Check sheet for the modelled part. Datum: model origin and axes. Units: mm. Face numbers are marked on the shaded views. Round coordinates to 2 decimals unless told otherwise and drop trailing zeros. Order: outer loops, then holes, each group sorted by start corner. A loop starts at its lowest first (then second) coordinate and runs counter-clockwise, first axis right, second up. Notation, with made-up numbers: M 53.25,-17.5 L 83.25,-17.5 A7 ccw 83.25,-8.5 Z; hole C -30,66.5 d3. An arc over 180 degrees is marked long. One line per item, written item: value. Start each with the question number.
(1) Release check for a two-part mould opening along Y. For the marked faces 1, 2 and 3 record: released by +Y, released by -Y, zero draft, split by the parting line, or undercut.
(2) Cross-section at B-B, the plane y = 31. Enter the section's corners in (x, z), and give its area (3 significant figures).
(3) Thickness scan on L1, parallel to Z at x = 0.05, y = 2; L2, parallel to Z at x = 0.4, y = 19.5; L3, parallel to X at y = 31.5, z = -0.35. Record the ranges inside material, lowest first.
(4) Cross-section at A-A, the plane y = 25. Enter the section's corners in (x, z).
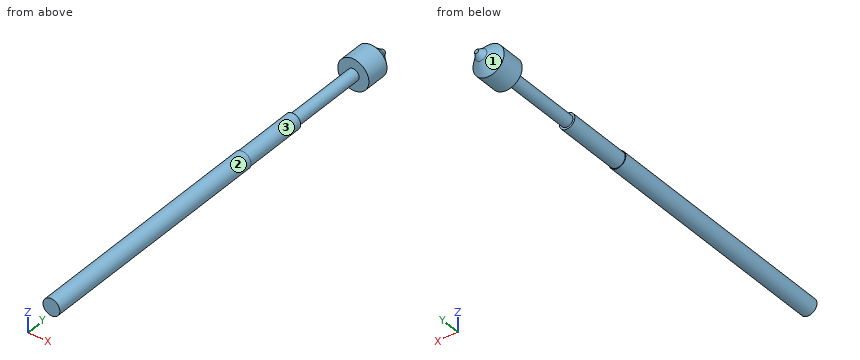
from build123d import *

# Parameters (mm, degrees)
SKETCH_1_R      = 0.65
EXTRUDE_1_DEPTH = 19
SKETCH_2_R      = 0.6
EXTRUDE_2_DEPTH = 5
SKETCH_3_R      = 0.45
EXTRUDE_3_DEPTH = 9


with BuildPart() as part:
    # 草图1 → 凸台-拉伸1 (new body)
    with BuildSketch(Plane(origin=(0, 0, 0), x_dir=(1, 0, 0), z_dir=(0, 1, 0))):
        with Locations(Location((0, 0, 0), (0, 0, 270))):
            Circle(SKETCH_1_R)
    extrude(amount=EXTRUDE_1_DEPTH)

    # 草图2 → 凸台-拉伸2 (add)
    with BuildSketch(Plane(origin=(0, 19, 0), x_dir=(1, 0, 0), z_dir=(0, 1, 0))):
        with Locations(Location((0, 0, 0), (0, 0, 270))):
            Circle(SKETCH_2_R)
    extrude(amount=EXTRUDE_2_DEPTH)

    # 草图3 → 凸台-拉伸3 (add)
    with BuildSketch(Plane(origin=(0, 24, 0), x_dir=(1, 0, 0), z_dir=(0, 1, 0))):
        with Locations(Location((0, 0, 0), (0, 0, 270))):
            Circle(SKETCH_3_R)
    extrude(amount=EXTRUDE_3_DEPTH)

    # 草图6 → 旋转2 (revolve)
    with BuildSketch(Plane.XY, mode=Mode.PRIVATE) as revolve_2_sk:
        Polygon((0, 33), (-1.2, 31.8), (-1.2, 30), (0, 30), align=None)
    revolve(revolve_2_sk.sketch.rotate(Axis((0, 0, 0), (0, -1, 0)), 180), axis=Axis((0, 0, 0), (0, -1, 0)))

    # 草图7 → 切除-旋转5 (revolve, cut)
    with BuildSketch(Plane.XY):
        Polygon((0.45, 33), (0.15, 33), (0.45, 32.55), align=None)
    revolve(axis=Axis((0, 0, 0), (0, -1, 0)), mode=Mode.SUBTRACT)


solid = part.part
Values found:
1. face 1: released by +Y
1. face 2: zero draft
1. face 3: undercut
2. outline: C 0,0 d2.4
2. area: 4.52 mm^2
3. L1: -0.65 to 0.65
3. L2: -0.45 to 0.45
3. L3: -1.15 to 1.15
4. outline: C 0,0 d0.9
